```python
from build123d import *

# Parameters (mm, degrees)
BOSS_EXTRUDE1_DEPTH = 6
SKETCH2_OUTSIDE_W   = 39.322
SKETCH2_OUTSIDE_H   = 36.654
SKETCH2_OUTSIDE_R   = 8.625
CUT_EXTRUDE1_DEPTH  = 6
CUT_EXTRUDE1_DRAFT  = -45
SKETCH3_OUTSIDE_W   = 39.322
SKETCH3_OUTSIDE_H   = 36.654
SKETCH3_OUTSIDE_R   = 8.625
CUT_EXTRUDE2_DEPTH  = 6
CUT_EXTRUDE2_DRAFT  = -45
SKETCH4_R           = 4.5
CUT_EXTRUDE3_DEPTH  = 7


with BuildPart() as part:
    # Sketch1 → Boss-Extrude1 (new body)
    with BuildSketch(Plane.XY):
        Polygon((9.959292144, 0), (4.979646072, 8.625), (-4.979646072, 8.625), (-9.959292144, 0), (-4.979646072, -8.625), (4.979646072, -8.625), align=None)
    extrude(amount=BOSS_EXTRUDE1_DEPTH)


with BuildPart() as cut_extrude1_tool:
    # Sketch2 outside → Cut-Extrude1 (with draft: the straight prism first)
    with BuildSketch(Plane.XY.offset(6)):
        Rectangle(SKETCH2_OUTSIDE_W, SKETCH2_OUTSIDE_H)
        Circle(SKETCH2_OUTSIDE_R, mode=Mode.SUBTRACT)
    extrude(amount=-CUT_EXTRUDE1_DEPTH)
    # Cut-Extrude1: the draft: its side faces are tilted about the plane it starts from
    cut_extrude1_sides = [cut_extrude1_tool.faces().sort_by_distance(p)[0] for p in [
        (0, -18.327, 3),
        (19.661, 0, 3),
        (0, 18.327, 3),
        (-19.661, 0, 3),
        (-8.625, 0, 3),
    ]]
    draft(cut_extrude1_sides, Plane.XY.offset(6), CUT_EXTRUDE1_DRAFT)


with BuildPart() as part_1:
    add(part.part)

    # Cut-Extrude1: cut by cut_extrude1_tool
    add(cut_extrude1_tool.part, mode=Mode.SUBTRACT)


with BuildPart() as cut_extrude2_tool:
    # Sketch3 outside → Cut-Extrude2 (with draft: the straight prism first)
    with BuildSketch(Plane(origin=(0, 0, 0), x_dir=(-1, 0, 0), z_dir=(0, 0, -1))):
        Rectangle(SKETCH3_OUTSIDE_W, SKETCH3_OUTSIDE_H)
        Circle(SKETCH3_OUTSIDE_R, mode=Mode.SUBTRACT)
    extrude(amount=-CUT_EXTRUDE2_DEPTH)
    # Cut-Extrude2: the draft: its side faces are tilted about the plane it starts from
    cut_extrude2_sides = [cut_extrude2_tool.faces().sort_by_distance(p)[0] for p in [
        (0, -18.327, 3),
        (-19.661, 0, 3),
        (0, 18.327, 3),
        (19.661, 0, 3),
        (8.625, 0, 3),
    ]]
    draft(cut_extrude2_sides, Plane(origin=(0, 0, 0), x_dir=(-1, 0, 0), z_dir=(0, 0, -1)), CUT_EXTRUDE2_DRAFT)


with BuildPart() as part_2:
    add(part_1.part)

    # Cut-Extrude2: cut by cut_extrude2_tool
    add(cut_extrude2_tool.part, mode=Mode.SUBTRACT)

    # Sketch4 → Cut-Extrude3 (cut, through all)
    with BuildSketch(Plane.XY.offset(6)):
        Circle(SKETCH4_R)
    extrude(amount=-CUT_EXTRUDE3_DEPTH, mode=Mode.SUBTRACT)


solid = part_2.part
```
Part model, mm, in its own coordinate system. Coordinates: 2 decimals unless noted, no trailing zeros. Order: outer loops, then holes, each group sorted by start corner. A loop starts at its lowest first (then second) coordinate and runs counter-clockwise, first axis right, second up. Notation, with made-up numbers: (-30.75, 0.5) -> (-1.75, 0.5) arc R25 ccw to (-1.75, 30.5) -> close; hole circle Ø10 at (-36.75, 67). An arc over 180 degrees is marked (long way). Put each result on its own line as item: value. Start each with the question number.
(1) Mould opens along Y. For faces 1 (the face through (-0.59, 4.46, 3.04)), 2 (the face through (4.45, -7.76, 5.68)), 3 (the face through (8.943, 0.022, 0.318)) say: pulls with the +Y half, pulls with the -Y half, needs draft (parallel to the pull), parting line crosses it, or undercut.
(2) Pin check, flat tip, straight feed: pin 1 Ø1.5 at (x, z) = (7.5, 3) entering from +Y. Stop position of the tip, or through.
(3) Probe line 1 along Y through (x, z) = (0, 4.7) (3 decimals); line 2 along X through (y, z) = (3, 4.55); line 3 along Y through (x, z) = (-1.5, 4.05) (3 decimals). List the from-to ranges inside material, lowest first. Write a range as [from, to].
(4) Band-saw the part on A-A (z = 2.95). Give the cut face in (x, y) (3 decimals).
Determined:
1. face 1: undercut
1. face 2: pulls with the -Y half
1. face 3: parting line crosses it
2. pin 1: stops at y = 5.56
3. line 1: y = [-8.625, -4.5], [4.5, 8.625]
3. line 2: x = [-8.23, -3.35], [3.35, 8.23]
3. line 3: y = [-8.625, -4.243], [4.243, 8.625]
4. outline: (-9.959, 0) -> (-4.98, -8.625) -> (4.98, -8.625) -> (9.959, 0) -> (4.98, 8.625) -> (-4.98, 8.625) -> close; hole circle Ø9 at (0, 0)
